For this review, take the finished solid that the model builds, in its own axes (mm). A direction names the side the tool comes from. Give positions to 0.01 mm unless a question says otherwise; leave off trailing zeros. Loops run counter-clockwise (first coordinate to the right, second up) from the corner with the lowest first, then second, coordinate; pieces in that order, holes last. Notation, with made-up numbers: (61.5, 71) - (119.5, 71) arc R11 ccw to (119.5, 85) - close; hole circle Ø7 at (-31.5, 89.25). An arc over 180 degrees is marked (long way). Put each result on its own line as item: value.
from build123d import *

# Parameters (mm, degrees)
F0_W           = 40
F0_H           = 120
F1_DEPTH       = 6
F3_D           = 5.5
F3_DEPTH       = 15
F3_CBORE_D     = 9.2
F3_CBORE_DEPTH = 3
F3_TIP         = 1.6523667023
F5_D           = 7
F5_DEPTH       = 15
F5_TIP         = 2.1030121666
F6_SIZE        = 5
F7_SIZE        = 2


# Not quite as in the source:
# - a pattern or mirror of a feature is missing from the dataset's text; its kind, count and spacing are read off the source's solid


with BuildPart() as f1:
    # F0 (on Top) → F1 (new body)
    with BuildSketch(Plane.XY):
        Rectangle(F0_W, F0_H)
    extrude(amount=F1_DEPTH)

    # F3
    with Locations(Plane.XY.offset(6)):
        with Locations((-13.875, 31.4), (13.875, 31.4), (-13.875, -31.4), (13.875, -31.4)):
            CounterBoreHole(F3_D / 2, F3_CBORE_D / 2, F3_CBORE_DEPTH, depth=F3_DEPTH)
            with Locations((0, 0, -(F3_DEPTH + F3_TIP / 2))):  # 118° drill point
                Cone(0, F3_D / 2, F3_TIP, mode=Mode.SUBTRACT)

    # F5
    with Locations(Plane.XY.offset(6)):
        with Locations((0, 47.5)):
            f5 = Hole(F5_D / 2, depth=F5_DEPTH)
            with Locations((0, 0, -(F5_DEPTH + F5_TIP / 2))):  # 118° drill point
                Cone(0, F5_D / 2, F5_TIP, mode=Mode.SUBTRACT)

    # F5_copies: F5 across plane
    add(f5.mirror(Plane(origin=(0, 0, 0), x_dir=(0, 0, -1), z_dir=(0, -1, 0))), mode=Mode.SUBTRACT)

    # F6
    f6_edges = [f1.edges().sort_by_distance(p)[0] for p in [
        (20, 60, 3),
        (-20, 60, 3),
        (-20, -60, 3),
        (20, -60, 3),
    ]]
    chamfer(f6_edges, length=F6_SIZE)

    # F7
    f7_edges = [f1.edges().sort_by_distance(p)[0] for p in [
        (0, 60, 0),
        (-17.5, 57.5, 0),
        (17.5, 57.5, 0),
        (17.5, -57.5, 0),
        (0, -60, 0),
        (-17.5, -57.5, 0),
    ]]
    chamfer(f7_edges, length=F7_SIZE)


solid = f1.part
1) Insertion check: pin 1 Ø11 at (x, y) = (0, -47.5) entering from +Z; pin 2 Ø4.5 at (x, y) = (13.875, 31.4) entering from -Z; pin 3 Ø3 at (x, y) = (-15, -30.5) entering from +Z. Each pin has a flat end and moves straight along its axis. Give the tip position at first contact, or say it passes through.
Geometry check:
pin 1: stops at z = 6
pin 2: passes through
pin 3: stops at z = 3
2) Take a section at A-A on y = 47.5. State the section outline as (x, z) points, and give its area (3 significant figures).
Geometry check:
outline: (-20, 0) - (-3.5, 0) - (-3.5, 6) - (-20, 6) - close; (3.5, 0) - (20, 0) - (20, 6) - (3.5, 6) - close
area: 198 mm²
3) Take a section at C-C on z = 5. State the section outline as (x, y) points (3 decimals).
Geometry check:
outline: (-20, -55) - (-15, -60) - (15, -60) - (20, -55) - (20, 55) - (15, 60) - (-15, 60) - (-20, 55) - close; hole circle Ø9.2 at (-13.875, -31.4); hole circle Ø9.2 at (-13.875, 31.4); hole circle Ø7 at (0, -47.5); hole circle Ø7 at (0, 47.5); hole circle Ø9.2 at (13.875, -31.4); hole circle Ø9.2 at (13.875, 31.4)
4) Draft analysis for pull direction X (two halves, no side actions). For faces 3 (the face through (17.46, 56.14, 1.01)), 4 (the face through (0, -59, 1)), 5 (the face through (16.06, -33.07, 1.48)), 6 (the face through (-12, 29, 3)), state which applies: pulls with the +X half, pulls with the -X half, needs draft (parallel to the pull), parting line crosses it, or undercut.
Geometry check:
face 3: pulls with the +X half
face 4: needs draft
face 5: undercut
face 6: undercut
5) Wall thickness on line 1 (Y direction, x = 0, z = 3.7); line 2 (Y direction, x = -14, z = 5); line 3 (X direction, y = -30, z = 3.75): over which ranges is each line inside the solid? List them lowest first.
Geometry check:
line 1: y = -60 to -51, -44 to 44, 51 to 60
line 2: y = -60 to -36, -26.8 to 26.8, 36 to 60
line 3: x = -20 to -18.26, -9.49 to 9.49, 18.26 to 20
6) Take a section at B-B on x = 0. State the section outline as (y, z) points, and give its area (3 significant figures).
Geometry check:
outline: (-60, 2) - (-58, 0) - (-51, 0) - (-51, 6) - (-60, 6) - close; (-44, 0) - (44, 0) - (44, 6) - (-44, 6) - close; (51, 0) - (58, 0) - (60, 2) - (60, 6) - (51, 6) - close
area: 632 mm²
7) Take a section at D-D on y = -31.4. State the section outline as (x, z) points (3 decimals).
Geometry check:
outline: (-20, 0) - (-16.625, 0) - (-16.625, 3) - (-18.475, 3) - (-18.475, 6) - (-20, 6) - close; (-11.125, 0) - (11.125, 0) - (11.125, 3) - (9.275, 3) - (9.275, 6) - (-9.275, 6) - (-9.275, 3) - (-11.125, 3) - close; (16.625, 0) - (20, 0) - (20, 6) - (18.475, 6) - (18.475, 3) - (16.625, 3) - close
8) For faces 1 (the face through (13.8, -34.4, 3)), 2 (the face through (0, 59, 1)), list the 3-axis set-ups (+Z, -Z, +X, -X, +Y, -Y) from which the entire face can be reached by the end or side of a thin tool; tool diameter is ignored.
Geometry check:
face 1: +Z
face 2: -Z, +X, -X, +Y
